Source: CAD feature listing. Evaluate the final solid. Frame: model axes, mm. Round coordinates to 2 decimals unless told otherwise and drop trailing zeros. Order: outer loops, then holes, each group sorted by start corner. A loop starts at its lowest first (then second) coordinate and runs counter-clockwise, first axis right, second up. Notation, with made-up numbers: M 28,65.5 L 65,65.5 A11 cw 65,73.5 Z; hole C -26,-20 d2. An arc over 180 degrees is marked long. Use one line per item in the form item = value. Start each with the question number.
Q1. Section D-D (z = 2.5). Return the cut outline in (x, y).
Q2. Section B-B (z = 10.5). Return the cut outline in (x, y).
Q3. Contact query for a flat-ended pin moving along its axis: pin 1 (5 mm diameter, centred on y = 3, z = 3, fed in from -X). Output: stop coordinate, or through.
Q4. Section C-C (y = 0). Return the cut outline in (x, z).
Q5. Section A-A (x = 19). Return the cut outline in (y, z).
Q6. Material intervals for probe 1 along X at (y, z) = (-6.5, 9.25); probe 2 along Y at (x, z) = (2.5, 1.75); probe 3 along Z at (x, y) = (19, 7.75), sorted ascending.
Q7. Pull-direction query (Z, two-part tool) for faces 1 (the cylindrical face through (10.526, -0.175, 11.852)), 2 (the flat face through (0, 0, 9)), 3 (the cylindrical face through (11.83, -0.16, 7.5)); classes: pulls with the +Z half, pulls with the -Z half, needs draft (parallel to the pull), parting line crosses it, or undercut.
Autodesk Inventor part; units mm, degrees
ref_plane "YZ Plane" through (0, 0, 0) normal (1, 0, 0) x (0, 1, 0)
ref_plane "XZ Plane" through (0, 0, 0) normal (0, 1, 0) x (-1, 0, 0)
ref_plane "XY Plane" through (0, 0, 0) normal (0, 0, 1) x (1, 0, 0)
sketch "Sketch1" plane through (0, 0, 0) normal (1, 0, 0) x (0, 1, 0)
  arc A0 (7.5, 0) -> (-7.5, 0) centre (0, 0) ccw
  line L0 (7.5, 0) -> (12.5, 0)
  line L1 (12.5, 0) -> (12.5, 15)
  line L2 (12.5, 15) -> (-12.5, 15)
  line L3 (-12.5, 15) -> (-12.5, 0)
  line L4 (-12.5, 0) -> (-7.5, 0)
  dimension "d0" = 15
  dimension "d1" = 12.5
  dimension "d2" = 15
  dimension "d3" = 25
extrude "Extrusion1" add sketch "Sketch1" along normal blind 24
sketch "Sketch2" plane through (0, -12.5, 0) normal (0, -1, 0) x (1, 0, 0)
  circle A0 centre (5, 10.5) radius 2
  circle A1 centre (12, 10.5) radius 2
  circle A2 centre (19, 10.5) radius 2
  dimension "d11" = 4
extrude "Extrusion2" cut sketch "Sketch2" against normal blind 25
properties part number "Y_RodClam_Bed" material "Birch"
Results list:
q1.outline = M 0,-12.5 L 24,-12.5 L 24,-7.07 L 0,-7.07 Z; M 0,7.07 L 24,7.07 L 24,12.5 L 0,12.5 Z
q2.outline = M 0,-12.5 L 3,-12.5 L 3,12.5 L 0,12.5 Z; M 7,-12.5 L 10,-12.5 L 10,12.5 L 7,12.5 Z; M 14,-12.5 L 17,-12.5 L 17,12.5 L 14,12.5 Z; M 21,-12.5 L 24,-12.5 L 24,12.5 L 21,12.5 Z
q3.pin_1 = through
q4.outline = M 0,7.5 L 24,7.5 L 24,15 L 0,15 Z; hole C 5,10.5 d4; hole C 12,10.5 d4; hole C 19,10.5 d4
q5.outline = M -12.5,0 L -7.5,0 A7.5 cw 7.5,0 L 12.5,0 L 12.5,8.5 L -12.5,8.5 Z; M -12.5,12.5 L 12.5,12.5 L 12.5,15 L -12.5,15 Z
q6.probe_1 = 0 to 3.44, 6.56 to 10.44, 13.56 to 17.44, 20.56 to 24
q6.probe_2 = -12.5 to -7.29, 7.29 to 12.5
q6.probe_3 = 0 to 8.5, 12.5 to 15
q7.face_1 = undercut
q7.face_2 = needs draft
q7.face_3 = pulls with the -Z half
